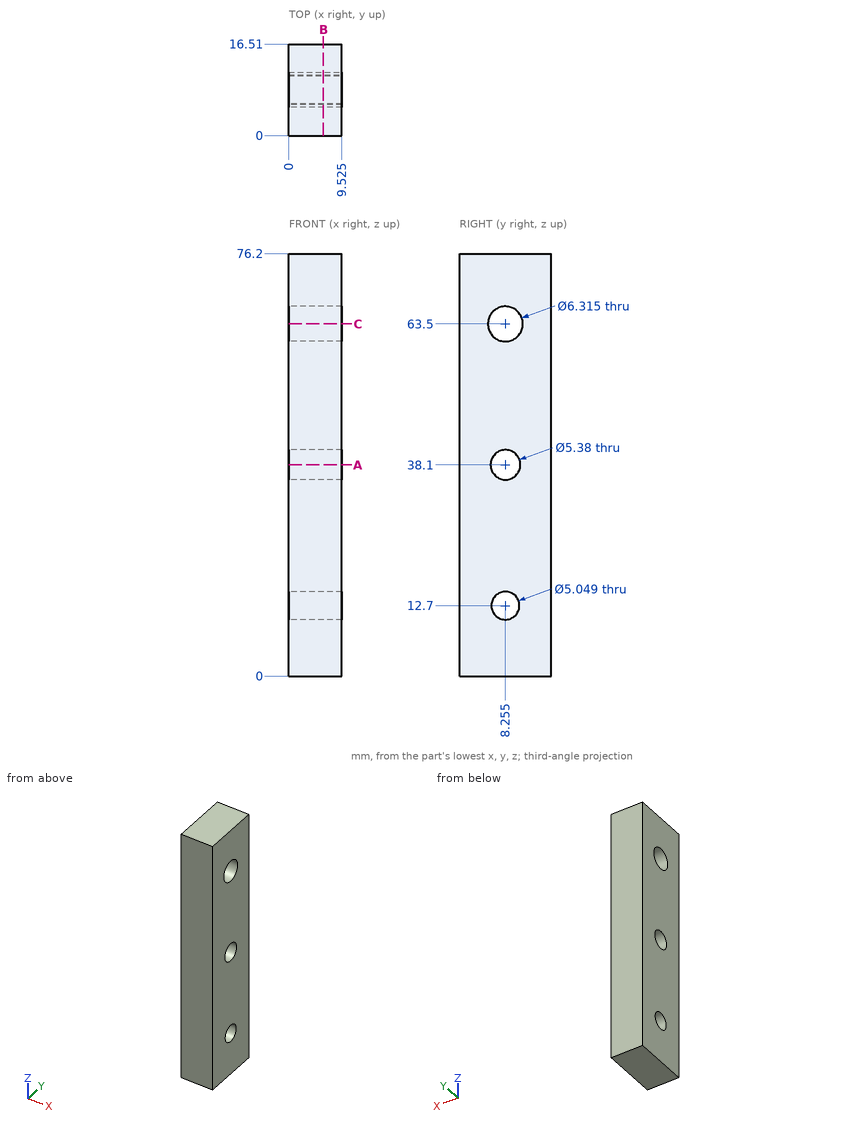
Could you check a few things on this drawing? It's one solid part, dimensions in mm from its lowest x, y, z. Give positions to 0.01 mm unless a question says otherwise; leave off trailing zeros. Order: outer loops, then holes, each group sorted by start corner. A loop starts at its lowest first (then second) coordinate and runs counter-clockwise, first axis right, second up. Notation, with made-up numbers: (61, -9) -> (81, -9) arc R13 ccw to (81, -4) -> close; hole circle Ø2 at (-24.75, 40.5). An arc over 180 degrees is marked (long way). Use CSV: the item, a comma, the result in double quotes. Start each with the question number.
Item 1: If I drill on probe 1 along Z at (x, y) = (9, 10) (1 decimal); probe 2 along Z at (x, y) = (2.75, 8.75) (1 decimal); probe 3 along Y at (x, z) = (8.75, 39), over which ranges is the centre line in solid material (lowest first)? Write a range as [from, to].
Item 2: Suppose I cut it at C-C (z = 63.5). List the corners of the cut face in (x, y) for me (1 decimal).
Item 3: Suppose I cut it at B-B (x = 6.25). List the corners of the cut face in (y, z) for me (1 decimal).
Item 4: I'm going to push a flat-ended pin straight in: P1, Ø3, axis at y = 8.255, z = 38.1, coming from the -X side. Where does the tip first touch, or does it pass through?
Item 5: Suppose I cut it at A-A (z = 38.1). List the corners of the cut face in (x, y) for me (1 decimal).
Answer block:
1,probe 1,"z = [0, 10.9], [14.5, 36.1], [40.1, 60.9], [66.1, 76.2]"
1,probe 2,"z = [0, 10.2], [15.2, 35.5], [40.7, 60.4], [66.6, 76.2]"
1,probe 3,"y = [0, 5.72], [10.79, 16.51]"
2,outline,"(0, 0) -> (9.5, 0) -> (9.5, 5.1) -> (0, 5.1) -> close; (0, 11.4) -> (9.5, 11.4) -> (9.5, 16.5) -> (0, 16.5) -> close"
3,outline,"(0, 0) -> (16.5, 0) -> (16.5, 76.2) -> (0, 76.2) -> close; hole circle Ø6.3 at (8.3, 63.5); hole circle Ø5.4 at (8.3, 38.1); hole circle Ø5 at (8.3, 12.7)"
4,P1,"passes through"
5,outline,"(0, 0) -> (9.5, 0) -> (9.5, 5.6) -> (0, 5.6) -> close; (0, 10.9) -> (9.5, 10.9) -> (9.5, 16.5) -> (0, 16.5) -> close"
